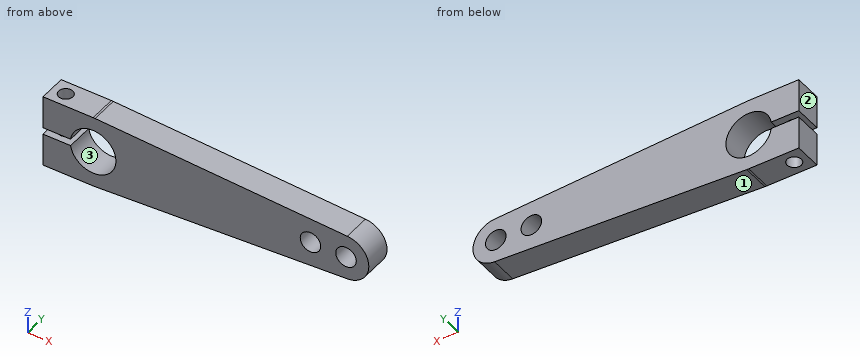
from build123d import *

# Parameters (mm, degrees)
CROQUIS1_R              = 10
SALIENTE_EXTRUIR1_DEPTH = 12
CROQUIS2_W              = 21.833325304
CROQUIS2_H              = 3
CORTAR_EXTRUIR1_DEPTH   = 12
CROQUIS3_R              = 3.125
CORTAR_EXTRUIR2_DEPTH   = 126.733845881
CORTAR_EXTRUIR3_REACH   = 124.642
CROQUIS6_R              = 4.5


with BuildPart() as part:
    # Croquis1 → Saliente-Extruir1 (new body)
    with BuildSketch(Plane(origin=(0, 0, 0), x_dir=(1, 0, 0), z_dir=(0, 1, 0))):
        with BuildLine():
            Line((0.864864865, 15.976608175), (111.540540541, 9.985380109))
            ThreePointArc((111.540540541, 9.985380109), (121, 0), (111.540540541, -9.985380109))
            Line((111.540540541, -9.985380109), (0.864864865, -15.976608175))
            ThreePointArc((0.864864865, -15.976608175), (0.432590572, -15.994150975), (0, -16))
            Line((0, -16), (-22, -16))
            Line((-22, -16), (-22, 16))
            Line((-22, 16), (0, 16))
            ThreePointArc((0, 16), (0.432590572, 15.994150975), (0.864864865, 15.976608175))
        make_face()
        with Locations(Location((0, 0, 0), (0, 0, 270))):
            Circle(CROQUIS1_R, mode=Mode.SUBTRACT)
    extrude(amount=SALIENTE_EXTRUIR1_DEPTH)

    # Croquis2 → Cortar-Extruir1 (cut)
    with BuildSketch(Plane(origin=(0, 12, 0), x_dir=(1, 0, 0), z_dir=(0, 1, 0))):
        with Locations((-17.033164983, 0)):
            Rectangle(CROQUIS2_W, CROQUIS2_H)
    extrude(amount=-CORTAR_EXTRUIR1_DEPTH, mode=Mode.SUBTRACT)

    # Croquis3 → Cortar-Extruir2 (cut, through all)
    with BuildSketch(Plane.XY.offset(16)):
        with Locations((-16, 6)):
            Circle(CROQUIS3_R)
    extrude(amount=-CORTAR_EXTRUIR2_DEPTH, mode=Mode.SUBTRACT)

    # Croquis6 → Cortar-Extruir3 (cut, up to next)
    with BuildSketch(Plane(origin=(0, 12, 0), x_dir=(1, 0, 0), z_dir=(0, 1, 0)), mode=Mode.PRIVATE) as cortar_extruir3_sk1:
        with Locations(Location((111, 0, 0), (0, 0, 270))):
            Circle(CROQUIS6_R)
    cortar_extruir3_tool1 = extrude(cortar_extruir3_sk1.sketch, amount=-CORTAR_EXTRUIR3_REACH, mode=Mode.PRIVATE) & part.part
    # Croquis6 → Cortar-Extruir3 (cut, up to next)
    with BuildSketch(Plane(origin=(0, 12, 0), x_dir=(1, 0, 0), z_dir=(0, 1, 0)), mode=Mode.PRIVATE) as cortar_extruir3_sk2:
        with Locations(Location((95.4, 0, 0), (0, 0, 270))):
            Circle(CROQUIS6_R)
    cortar_extruir3_tool2 = extrude(cortar_extruir3_sk2.sketch, amount=-CORTAR_EXTRUIR3_REACH, mode=Mode.PRIVATE) & part.part
    add(cortar_extruir3_tool1.solids().sort_by_distance((111, 12, 0))[0], mode=Mode.SUBTRACT)
    add(cortar_extruir3_tool2.solids().sort_by_distance((95.4, 12, 0))[0], mode=Mode.SUBTRACT)


solid = part.part
Can you work these out from the model? Positions are in its coordinate system, mm. Face numbers are marked on the shaded views. Round coordinates to 2 decimals unless told otherwise and drop trailing zeros. Write each loop counter-clockwise with the first axis right and the second up, starting at its lowest first coordinate (ties: lowest second). Pieces come first, ordered by that corner, then holes. Notation, with made-up numbers: (85.25, -37.75) -> (102.25, -37.75) arc R20 ccw to (102.25, -1.75) -> close; hole circle Ø3 at (46.25, -34). An arc over 180 degrees is marked (long way). Use one line per item in the form item = value. Start each with the question number.
Q1. Imagine slicing it at B-B (x = -16). Please give me the cut outline in (y, z) (3 decimals).
Q2. If I drill on probe 1 along X at (y, z) = (4.75, 0); probe 2 along Z at (x, y) = (-12.5, 9.5); probe 3 along Y at (x, z) = (-16, 6) (3 decimals), over which ranges is the centre line in solid material (lowest first)? Write a range as [from, to].
Q3. Imagine slicing it at C-C (y = 6). Please give me the cut outline in (x, z) (3 decimals), then the cut area to 3 significant figures.
Q4. I'm going to push flat-ended pins straight in: P1, Ø1.5, axis at x = 1, y = 4, coming from the +Z side; P2, Ø1.5, axis at x = 34.5, y = 7, coming from the +Z side. Where does each tip first touch, or does it pass through?
Q5. Imagine slicing it at A-A (z = 0). Please give me the cut outline in (x, y).
Q6. We'd pull the mould along Z, two halves only. Please class the marked faces 1, 2 and 3: +Z half, -Z half, draft (parallel to the pull), parting line (faces both ways), or undercut.
Q7. Imagine slicing it at D-D (z = -8). Please give me the cut outline in (x, y) (3 decimals), then the cut area to 3 significant figures.
Worked out:
q1.outline = (0, -16) -> (2.875, -16) -> (2.875, -1.5) -> (0, -1.5) -> close; (0, 1.5) -> (2.875, 1.5) -> (2.875, 16) -> (0, 16) -> close; (9.125, -16) -> (12, -16) -> (12, -1.5) -> (9.125, -1.5) -> close; (9.125, 1.5) -> (12, 1.5) -> (12, 16) -> (9.125, 16) -> close
q2.probe_1 = [10, 90.9], [99.9, 106.5], [115.5, 121]
q2.probe_2 = [-16, -1.5], [1.5, 16]
q2.probe_3 = [0, 2.875], [9.125, 12]
q3.outline = (-22, -16) -> (-19.125, -16) -> (-19.125, -1.5) -> (-22, -1.5) -> close; (-22, 1.5) -> (-19.125, 1.5) -> (-19.125, 16) -> (-22, 16) -> close; (-12.875, -16) -> (0, -16) arc R16 ccw to (0.865, -15.977) -> (111.541, -9.985) arc R10 ccw to (111.541, 9.985) -> (0.865, 15.977) arc R16 ccw to (0, 16) -> (-12.875, 16) -> (-12.875, 1.5) -> (-9.887, 1.5) arc R10 cw (long way) to (-9.887, -1.5) -> (-12.875, -1.5) -> close; hole circle Ø9 at (95.4, 0); hole circle Ø9 at (111, 0)
q3.area = 3,090 mm^2
q4.P1 = 16
q4.P2 = 14.2
q5.outline = (10, 0) -> (90.9, 0) -> (90.9, 12) -> (10, 12) -> close; (99.9, 0) -> (106.5, 0) -> (106.5, 12) -> (99.9, 12) -> close; (115.5, 0) -> (121, 0) -> (121, 12) -> (115.5, 12) -> close
q6.face_1 = -Z half
q6.face_2 = draft
q6.face_3 = undercut
q7.outline = (-22, 0) -> (-6, 0) -> (-6, 12) -> (-22, 12) -> close; (6, 0) -> (117, 0) -> (117, 12) -> (6, 12) -> close; hole circle Ø6.25 at (-16, 6)
q7.area = 1,490 mm^2
